Part model, mm, in its own coordinate system. A direction names the side the tool comes from. Coordinates: 2 decimals unless noted, no trailing zeros. Loops run counter-clockwise (first coordinate to the right, second up) from the corner with the lowest first, then second, coordinate; pieces in that order, holes last. Notation, with made-up numbers: M 22,-2.75 L 70,-2.75 A18 cw 70,18.25 Z; hole C 86.25,3 d9. An arc over 180 degrees is marked long. Use a Markdown table: item, result. Add a question column.
1) Pin check, flat tips, straight feed: pin 1 Ø1.5 at (x, z) = (24.5, 2) entering from +Y; pin 2 Ø6 at (x, z) = (32.5, -2.5) entering from +Y; pin 3 Ø4 at (y, z) = (-10, -8.5) entering from +X. Stop position of each tip, or through.
2) Wall check: probe 1 along X at (y, z) = (4, 15); probe 2 along Y at (x, z) = (72, 0); probe 3 along Z at (x, y) = (35, -0.5). Give the ranges that are in metal, low to high. Write a range as from..to.
3) Band-saw the part on A-A (x = 42.5). List the corners of the cut face in (y, z), plus the area to 3 significant figures.
4) Tool access for faces 1 (the conical face through (1.046, 13.958, -14.061)), 2 (the flat face through (15, 0.3, 12.3)): list every direction of +Z, -Z, +X, -X, +Y, -Y with a clear straight run to the whole face (end or side of a thin tool).
from build123d import *

# Parameters (mm, degrees)
SKETCH1_W      = 36
SKETCH1_H      = 36
BASEHEAD_DEPTH = 15


with BuildPart() as part:
    # Sketch1 → BaseHead (new body)
    with BuildSketch(Plane(origin=(0, 0, 0), x_dir=(0, 0, -1), z_dir=(1, 0, 0))):
        Rectangle(SKETCH1_W, SKETCH1_H)
    extrude(amount=BASEHEAD_DEPTH)

    # BodySke → BaseBody (revolve)
    with BuildSketch(Plane.XY, mode=Mode.PRIVATE) as basebody_sk:
        Polygon((0, 0), (115, 0), (115, 10.352), (113.352, 12), (0, 12), align=None)
    revolve(basebody_sk.sketch.rotate(Axis((0, 0, 0), (1, 0, 0)), 90), axis=Axis((0, 0, 0), (1, 0, 0)))

    # Sketch3 → HeadChamfer (revolve, cut)
    with BuildSketch(Plane.XY):
        Polygon((0, 18), (5.196152423, 27), (5.196152423, 28), (-1, 28), (-1, 18), align=None)
    revolve(axis=Axis((0, 0, 0), (1, 0, 0)), mode=Mode.SUBTRACT)


solid = part.part
Entries:
| question | item | result |
|---|---|---|
| 1 | pin 1 | y = 11.93 |
| 1 | pin 2 | y = 12 |
| 1 | pin 3 | x = 114.23 |
| 2 | probe 1 | 0..15 |
| 2 | probe 2 | -12..12 |
| 2 | probe 3 | -11.99..11.99 |
| 3 | outline | C 0,0 d24 |
| 3 | area | 452 mm2 |
| 4 | face 1 | -Z, -X, +Y |
| 4 | face 2 | +X |
